Geometry check sheet. Reference: the model listing, model coordinates, mm. A direction names the side the tool comes from. Coordinates: 2 decimals unless noted, no trailing zeros. Write each loop counter-clockwise with the first axis right and the second up, starting at its lowest first coordinate (ties: lowest second). Pieces come first, ordered by that corner, then holes. Notation, with made-up numbers: (29, 8.25) -> (60, 8.25) arc R32 ccw to (60, 37.25) -> close; hole circle Ø4 at (-22, 55). An arc over 180 degrees is marked (long way). Answer as CSV lines item,"result".
```python
from build123d import *

# Parameters (mm, degrees)
BOSS_EXTRUDE1_DEPTH = 0.75
BOSS_EXTRUDE2_DEPTH = 13.5
SKETCH4_W           = 20
SKETCH4_H           = 20
BOSS_EXTRUDE3_DEPTH = 0.75
BOSS_EXTRUDE7_DEPTH = 3
CUT_EXTRUDE1_DEPTH  = 32.340867888


with BuildPart() as part:
    # Sketch1 → Boss-Extrude1 (new body)
    with BuildSketch(Plane(origin=(0, 0, 0), x_dir=(1, 0, 0), z_dir=(0, 1, 0))):
        Polygon((0, 0), (0, 20), (4.25, 20), (4.25, 4.25), (20, 4.25), (20, 0), align=None)
    extrude(amount=BOSS_EXTRUDE1_DEPTH)

    # Sketch2 → Boss-Extrude2 (add)
    with BuildSketch(Plane(origin=(0, 0.75, 0), x_dir=(1, 0, 0), z_dir=(0, 1, 0))):
        Polygon((20, 3.5), (20, 4.25), (4.25, 4.25), (4.25, 20), (3.5, 20), (3.5, 3.5), align=None)
        Polygon((0.75, 20), (0, 20), (0, 0), (20, 0), (20, 0.75), (0.75, 0.75), align=None)
    extrude(amount=BOSS_EXTRUDE2_DEPTH)

    # Sketch4 → Boss-Extrude3 (add)
    with BuildSketch(Plane.XZ):
        with Locations((10, -10)):
            Rectangle(SKETCH4_W, SKETCH4_H)
    extrude(amount=-BOSS_EXTRUDE3_DEPTH)

    # Sketch7 → Boss-Extrude7 (add)
    with BuildSketch(Plane.XZ):
        Polygon((0, 0), (0, -20), (0.75, -20), (0.75, -0.75), (20, -0.75), (20, 0), align=None)
    extrude(amount=BOSS_EXTRUDE7_DEPTH)

    # Sketch8 → Cut-Extrude1 (cut, through all)
    with BuildSketch(Plane(origin=(0, 0.75, 0), x_dir=(1, 0, 0), z_dir=(0, 1, 0))):
        Polygon((20, 4.25), (20, 20), (4.25, 20), align=None)
    extrude(amount=-CUT_EXTRUDE1_DEPTH, mode=Mode.SUBTRACT)


solid = part.part
```
Item 1: Thickness scan on probe 1 along X at (y, z) = (13.25, -9); probe 2 along Z at (x, y) = (3.75, 9.25); probe 3 along Z at (x, y) = (16.5, 13). Record the ranges inside material, lowest first.
Responses:
probe 1,"x = 0 to 0.75, 3.5 to 4.25"
probe 2,"z = -20 to -3.5, -0.75 to 0"
probe 3,"z = -4.25 to -3.5, -0.75 to 0"
Item 2: Set-up check for faces 4 (the flat face through (3.5, 7, -12)), 5 (the flat face through (8, 0, -8)), 6 (the flat face through (10, 0.75, -10)): record each of +Z, -Z, +X, -X, +Y, -Y from which the full face is reachable in a straight line by a thin tool's end or side.
Responses:
face 4,"-Z, +Y"
face 5,"-Z, +X, -Y"
face 6,"-Z, +X, +Y"
Item 3: Cross-section at B-B, the plane z = -15.5. Record the cut outline in (x, y).
Responses:
outline,"(0, -3) -> (0.75, -3) -> (0.75, 0) -> (8.75, 0) -> (8.75, 0.75) -> (4.25, 0.75) -> (4.25, 14.25) -> (3.5, 14.25) -> (3.5, 0.75) -> (0.75, 0.75) -> (0.75, 14.25) -> (0, 14.25) -> close"
Item 4: Release check for a two-part mould opening along X. For faces 1 (the flat face through (0.75, -1, -11)), 2 (the flat face through (3, 0.75, -7)), 3 (the flat face through (12, 7, -3.5)) record: +X half, -X half, draft (parallel to the pull), parting line (faces both ways), or undercut.
Responses:
face 1,"+X half"
face 2,"undercut"
face 3,"draft"
Item 5: Cross-section at C-C, the plane x = 19.25. Record the cut outline in (y, z).
Responses:
outline,"(-3, -0.75) -> (0, -0.75) -> (0, -5) -> (0.75, -5) -> (0.75, -4.25) -> (14.25, -4.25) -> (14.25, -3.5) -> (0.75, -3.5) -> (0.75, -0.75) -> (14.25, -0.75) -> (14.25, 0) -> (-3, 0) -> close"
Item 6: Depth check by flat-ended pin: pin 1 Ø7 at (x, y) = (14, 5) entering from +Z; pin 2 Ø6 at (x, z) = (16, -14) entering from +Y; pin 3 Ø4.5 at (x, z) = (13.5, -11) entering from +Y; pin 4 Ø1.5 at (y, z) = (-1.5, -8) entering from +X. Enter the tip coordinate at first touch or a pass-through.
Responses:
pin 1,"stops at z = 0"
pin 2,"passes through"
pin 3,"stops at y = 0.75"
pin 4,"stops at x = 0.75"
Item 7: Cross-section at D-D, the plane x = 3. Record the cut outline in (y, z), plus the area to 3 significant figures.
Responses:
outline,"(-3, -0.75) -> (0, -0.75) -> (0, -20) -> (0.75, -20) -> (0.75, -0.75) -> (14.25, -0.75) -> (14.25, 0) -> (-3, 0) -> close"
area,"27.4 mm2"
Item 8: Cross-section at A-A, the plane y = 4. Record the cut outline in (x, z), plus the area to 3 significant figures.
Responses:
outline,"(0, -20) -> (0.75, -20) -> (0.75, -0.75) -> (20, -0.75) -> (20, 0) -> (0, 0) -> close; (3.5, -20) -> (4.25, -20) -> (4.25, -4.25) -> (20, -4.25) -> (20, -3.5) -> (3.5, -3.5) -> close"
area,"53.6 mm2"
